from build123d import *

# Parameters (mm, degrees)
AUFSATZ_LINEAR_AUSTRAGEN2_DEPTH      = 20
VERRUNDUNG1_R                        = 15
SCHNITT_LINEAR_AUSTRAGEN3_DEPTH      = 229.701880893
SCHNITT_LINEAR_AUSTRAGEN3_DEPTH_BACK = 229.701880893
SKIZZE5_OUTSIDE_W                    = 521.679
SKIZZE5_OUTSIDE_H                    = 109.418
SCHNITT_LINEAR_AUSTRAGEN6_DEPTH      = 228.676613663
SKIZZE7_R                            = 17.5
SCHNITT_LINEAR_AUSTRAGEN5_DEPTH      = 0.1
SCHNITT_LINEAR_START                 = -0.1
SKIZZE9_R                            = 17.5
SCHNITT_LINEAR_AUSTRAGEN7_DEPTH      = 0.1
VERRUNDUNG5_R                        = 15


with BuildPart() as part:
    # Skizze1 → Aufsatz-Linear austragen2 (new body)
    with BuildSketch(Plane.XY):
        with BuildLine():
            Line((-216.718948666, 31.869537692), (-187.741173877, 24.104966339))
            ThreePointArc((-187.741173877, 24.104966339), (-188.20309721, 8.699595617), (-195.50574523, -4.87280845))
            Line((-195.50574523, -4.87280845), (-224.483520019, 2.891762903))
            ThreePointArc((-224.483520019, 2.891762903), (-199.032056143, -18.892233896), (-165.581524585, -17.053356943))
            Line((-165.581524585, -17.053356943), (-161.471528727, -11.5))
            Line((-161.471528727, -11.5), (150, -11.5))
            Line((150, -11.5), (177.209748999, -21.403538717))
            ThreePointArc((177.209748999, -21.403538717), (207.777170155, 0), (177.209748999, 21.403538717))
            Line((177.209748999, 21.403538717), (150, 11.5))
            Line((150, 11.5), (-150, 11.5))
            Line((-150, 11.5), (-155.735764364, 19.691520443))
            ThreePointArc((-155.735764364, 19.691520443), (-183.785335986, 38.009300378), (-216.718948666, 31.869537692))
        make_face()
    extrude(amount=AUFSATZ_LINEAR_AUSTRAGEN2_DEPTH)

    # Verrundung1
    verrundung1_edges = [part.edges().sort_by_distance(p)[0] for p in [
        (-150, 11.5, 10),
        (150, 11.5, 10),
        (150, -11.5, 10),
    ]]
    fillet(verrundung1_edges, radius=VERRUNDUNG1_R)

    # Skizze5 outside → Schnitt-Linear austragen3 (cut, two sides: drawn at the far end of the back side and taken through both)
    with BuildSketch(Plane(origin=(0, 0, 0), x_dir=(1, 0, 0), z_dir=(0, 1, 0)).offset(-SCHNITT_LINEAR_AUSTRAGEN3_DEPTH_BACK)):
        with Locations((-8.3535, -10)):
            Rectangle(SKIZZE5_OUTSIDE_W, SKIZZE5_OUTSIDE_H)
        Polygon((147.355095289, -15.5), (150.355095289, -18.5), (207.777170155, -17), (207.777170155, 0), (150.355095289, -1.5), (147.355095289, -4.5), (-142.191494242, -4.5), (-154.478774906, -3.5), (-224.483520019, -3.5), (-224.483520019, -16.5), (-154.478774906, -16.5), (-142.191494242, -15.5), align=None, mode=Mode.SUBTRACT)
    extrude(amount=SCHNITT_LINEAR_AUSTRAGEN3_DEPTH + SCHNITT_LINEAR_AUSTRAGEN3_DEPTH_BACK, mode=Mode.SUBTRACT)

    # Skizze8 → Schnitt-Linear austragen6 (cut, through all)
    with BuildSketch(Plane(origin=(-1.278585019, 0, 22.46102929), x_dir=(0.9996589857202393, 0, -0.026113449959408383), z_dir=(0.026113449959408383, 0, 0.9996589857202393))):
        Polygon((201.871273052, 0), (199.790762428, 7.764571353), (194.106701699, 13.448632083), (186.342130346, 15.529142706), (178.577558993, 13.448632083), (172.893498263, 7.764571353), (170.81298764, 0), (172.893498263, -7.764571353), (178.577558993, -13.448632083), (186.342130346, -15.529142706), (194.106701699, -13.448632083), (199.790762428, -7.764571353), align=None)
    extrude(amount=-SCHNITT_LINEAR_AUSTRAGEN6_DEPTH, mode=Mode.SUBTRACT)

    # Skizze7 → Schnitt-Linear austragen5 (cut)
    with BuildSketch(Plane(origin=(-0.373956847, 0, 5.437398269), x_dir=(-0.9996589857202394, 0, 0.026113449959408383), z_dir=(-0.026113449959408383, 0, -0.9996589857202394))):
        with Locations((-184.993264929, 0)):
            Circle(SKIZZE7_R)
    extrude(amount=-SCHNITT_LINEAR_AUSTRAGEN5_DEPTH, mode=Mode.SUBTRACT)

    # Skizze9 → Schnitt-Linear austragen7 (cut)
    with BuildSketch(Plane(origin=(0.585463065, 0, 22.412335959), x_dir=(0.9996589857202393, 0, -0.026113449959408383), z_dir=(0.026113449959408383, 0, 0.9996589857202393)).offset(SCHNITT_LINEAR_START)):
        with Locations(Location((184.477446379, 0, 0), (0, 0, 180))):
            Circle(SKIZZE9_R)
    extrude(amount=SCHNITT_LINEAR_AUSTRAGEN7_DEPTH, mode=Mode.SUBTRACT)

    # Verrundung5
    # the kernel refuses this fillet: 15 mm, written as the material it adds along each edge
    with BuildSketch(Plane(origin=(-161.471528727, -11.5, 3.5), x_dir=(1, 0, 0), z_dir=(0, 0, 1))) as verrundung5_piece_1_section:
        with BuildLine():
            CenterArc((7.541653594, -15), VERRUNDUNG5_R, 90, 50.96638681)
            Line((-4.109995858, -5.553356943), (-4.343028847, -5.364424082))
            ThreePointArc((-4.343028847, -5.364424082), (-2.296139873, -2.598211212), (-0.241141944, 0.178467259))
            Line((-0.241141944, 0.178467259), (0, 0.3))
            Line((0, 0.3), (7.541653594, 0.3))
            Line((7.541653594, 0.3), (7.541653594, 0))
        make_face()
    verrundung5_piece_1 = extrude(amount=13, mode=Mode.PRIVATE)
    verrundung5_piece_1 = split(verrundung5_piece_1, bisect_by=Plane(origin=(-154.879802837, -11.415872576, 16.532637647), z_dir=(-0.08111677690648599, 0, -0.9967046044361908)), keep=Keep.TOP, mode=Mode.PRIVATE)
    verrundung5_piece_1 = split(verrundung5_piece_1, bisect_by=Plane(origin=(-154.879802837, -11.415872576, 3.467362353), z_dir=(-0.08111677690648603, 0, 0.9967046044361908)), keep=Keep.TOP, mode=Mode.PRIVATE)
    add(verrundung5_piece_1)


solid = part.part
Design review of the part built by this model. Coordinates are the model's own, in mm. A direction names the side the tool comes from. Round coordinates to 2 decimals unless told otherwise and drop trailing zeros. Write each loop counter-clockwise with the first axis right and the second up, starting at its lowest first coordinate (ties: lowest second). Pieces come first, ordered by that corner, then holes. Notation, with made-up numbers: (-1, 72) - (58, 72) arc R25 cw to (58, 89) - close; hole circle Ø1 at (79, 87.25). An arc over 180 degrees is marked (long way). Use a Markdown table: item, result. Add a question column.
1. For faces 1 (the face through (-5, -11.5, 10)), 2 (the face through (-209.792, -1.045, 9.909)), 3 (the face through (-149.03, 13.15, 10.09)), list the 3-axis set-ups (+Z, -Z, +X, -X, +Y, -Y) from which the entire face can be reached by the end or side of a thin tool; tool diameter is ignored.
2. Clearance check with flat-ended pins moving along their axes: pin 1 (18.5 mm diameter, centred on x = 10, y = 1.5, fed in from +Z); pin 2 (4 mm diameter, centred on x = -77.5, z = 8.5, fed in from -Y); pin 3 (12 mm diameter, centred on x = 161.5, y = -7, fed in from +Z). State where each tip first meets the part, or that it passes through.
3. Mouldability with a two-part tool opening along Y and no side actions: class faces 4 (the face through (207.77, -0.61, 8.77)), 5 (the face through (5, 11.5, 10)), 6 (the face through (-202.43, 28.04, 9.91)) as +Y half, -Y half, draft (parallel to the pull), parting line (faces both ways), or undercut.
4. We need section A-A (x = -106). State the section outline as (y, z) points.
5. Wall thickness on probe 1 along Z at (x, y) = (-142.5, 6); probe 2 along Z at (x, y) = (-163.5, 26.5); probe 3 along Y at (x, z) = (183.5, 11): over which ranges is each line inside the solid? List them lowest first.
Output:
| question | item | result |
|---|---|---|
| 1 | face 1 | +Z, -Z, -Y |
| 1 | face 2 | +Z, -Z |
| 1 | face 3 | +Z, -Z, +Y |
| 2 | pin 1 | stops at z = 15.5 |
| 2 | pin 2 | stops at y = -11.5 |
| 2 | pin 3 | stops at z = 18.37 |
| 3 | face 4 | parting line |
| 3 | face 5 | +Y half |
| 3 | face 6 | undercut |
| 4 | outline | (-11.5, 4.5) - (11.5, 4.5) - (11.5, 15.5) - (-11.5, 15.5) - close |
| 5 | probe 1 | z = 4.47 to 15.53 |
| 5 | probe 2 | z = 3.5 to 16.5 |
| 5 | probe 3 | y = -22.73 to -15.17, 15.17 to 22.73 |
